from build123d import *

# Parameters (mm, degrees)
SKETCH1_W           = 93.98
SKETCH1_H           = 66.04
SKETCH1_W_2         = 83.82
SKETCH1_H_2         = 55.88
BOSS_EXTRUDE1_DEPTH = 27.08
SKETCH3_W           = 83.82
SKETCH3_H           = 55.88
BOSS_EXTRUDE2_DEPTH = 22
BOSS_EXTRUDE3_DEPTH = 10
FILLET1_R           = 2.54


with BuildPart() as part:
    # Sketch1 → Boss-Extrude1 (new body)
    with BuildSketch(Plane(origin=(0, 0, 0), x_dir=(1, 0, 0), z_dir=(0, 1, 0))):
        Rectangle(SKETCH1_W, SKETCH1_H)
        Rectangle(SKETCH1_W_2, SKETCH1_H_2, mode=Mode.SUBTRACT)
    extrude(amount=BOSS_EXTRUDE1_DEPTH)

    # Sketch3 → Boss-Extrude2 (add)
    with BuildSketch(Plane(origin=(0, 0, 0), x_dir=(1, 0, 0), z_dir=(0, 1, 0))):
        Rectangle(SKETCH3_W, SKETCH3_H)
    extrude(amount=BOSS_EXTRUDE2_DEPTH)

    # Sketch4 → Boss-Extrude3 (add)
    with BuildSketch(Plane.XZ):
        with BuildLine():
            Line((-30.48, 25.4), (30.48, 25.4))
            ThreePointArc((30.48, 25.4), (31.75, 24.13), (30.48, 22.86))
            Line((30.48, 22.86), (-30.48, 22.86))
            ThreePointArc((-30.48, 22.86), (-31.75, 24.13), (-30.48, 25.4))
        make_face()
    extrude(amount=BOSS_EXTRUDE3_DEPTH)

    # Fillet1
    fillet1_edges = [part.edges().sort_by_distance(p)[0] for p in [
        (46.99, 27.08, 0),
        (0, 27.08, -33.02),
        (-46.99, 27.08, 0),
        (0, 0, -33.02),
        (46.99, 0, 0),
        (0, 0, 33.02),
        (-46.99, 0, 0),
        (-46.99, 13.54, -33.02),
        (46.99, 13.54, -33.02),
        (46.99, 13.54, 33.02),
        (-46.99, 13.54, 33.02),
        (0, 27.08, 33.02),
    ]]
    fillet(fillet1_edges, radius=FILLET1_R)


solid = part.part
Model file for the job. Use its own axes, mm. A direction names the side the tool comes from. Give positions to 0.01 mm unless a question says otherwise; leave off trailing zeros. Order: outer loops, then holes, each group sorted by start corner. A loop starts at its lowest first (then second) coordinate and runs counter-clockwise, first axis right, second up. Notation, with made-up numbers: (-29, -19.5) - (2, -19.5) arc R26 ccw to (2, -5.5) - close; hole circle Ø1 at (21.25, 53.25). An arc over 180 degrees is marked (long way). Write item = value, one per line. Start each with the question number.
1. Cut at C-C, the plane y = -4.5. List the corners of the cut face in (x, z), and give its area (3 significant figures).
2. Drop flat-ended pins along their axis: P1, Ø8, axis at x = 7.5, y = -5.5, coming from the -Z side; P2, Ø5, axis at x = -13, y = -7.5, coming from the +Z side; P3, Ø2, axis at x = 11.5, z = -14.5, coming from the +Y side. Give the stop position or say it passes through.
3. Probe line 1 along Y through (x, z) = (-19.5, -6); line 2 along Z through (x, y) = (-13.5, -1.5); line 3 along Y through (x, z) = (-34.5, 30). List the from-to ranges inside material, lowest first.
4. Which spindle directions (+Z, -Z, +X, -X, +Y, -Y) get a long thin tool onto all of the face, cutting with end or side? Do faces 1 (the flat face through (-1, 25, 27.94)), 2 (the cylindrical face through (46.266, 26.316, -0.427)), 3 (the cylindrical face through (-31.75, -4.93, 24.1)), 4 (the flat face through (0, -5, 22.86)). Say none if no direction does.
5. Two-plate mould, pull along X, no slides. Class faces 5 (the flat face through (41.91, 25, 0)), 6 (the cylindrical face through (-46.266, 13.694, 32.256)), 7 (the flat face through (0, -5, 25.4)): pulls with the +X half, pulls with the -X half, needs draft (parallel to the pull), parting line crosses it, or undercut.
6. Cut at B-B, the plane z = 24.13. List the corners of the cut face in (x, y).
7. Cut at A-A, the plane x = 33.5. List the corners of the cut face in (y, z).
8. Cut at D-D, the plane z = -22.5. List the corners of the cut face in (x, y).
Taken from the geometry:
q1.outline = (-30.48, 22.86) - (30.48, 22.86) arc R1.27 ccw to (30.48, 25.4) - (-30.48, 25.4) arc R1.27 ccw to start
q1.area = 160 mm²
q2.P1 = 22.86
q2.P2 = 25.4
q2.P3 = 22
q3.line_1 = 0 to 22
q3.line_2 = 22.86 to 25.4
q3.line_3 = 0 to 27.08
q4.face_1 = +Y
q4.face_2 = +Z, -Z, +X, +Y
q4.face_3 = -X, -Y
q4.face_4 = -Z, +X, -X, -Y
q5.face_5 = undercut
q5.face_6 = pulls with the -X half
q5.face_7 = needs draft
q6.outline = (-46.99, 2.54) arc R2.54 ccw to (-44.45, 0) - (-31.75, 0) - (-31.75, -10) - (31.75, -10) - (31.75, 0) - (44.45, 0) arc R2.54 ccw to (46.99, 2.54) - (46.99, 24.54) arc R2.54 ccw to (44.45, 27.08) - (41.91, 27.08) - (41.91, 22) - (-41.91, 22) - (-41.91, 27.08) - (-44.45, 27.08) arc R2.54 ccw to (-46.99, 24.54) - close
q7.outline = (0, -30.48) arc R2.54 ccw to (2.54, -33.02) - (24.54, -33.02) arc R2.54 ccw to (27.08, -30.48) - (27.08, -27.94) - (22, -27.94) - (22, 27.94) - (27.08, 27.94) - (27.08, 30.48) arc R2.54 ccw to (24.54, 33.02) - (2.54, 33.02) arc R2.54 ccw to (0, 30.48) - close
q8.outline = (-46.99, 2.54) arc R2.54 ccw to (-44.45, 0) - (44.45, 0) arc R2.54 ccw to (46.99, 2.54) - (46.99, 24.54) arc R2.54 ccw to (44.45, 27.08) - (41.91, 27.08) - (41.91, 22) - (-41.91, 22) - (-41.91, 27.08) - (-44.45, 27.08) arc R2.54 ccw to (-46.99, 24.54) - close
